Work out the finished part from the listing and answer in its coordinate system (mm). A direction names the side the tool comes from. Give positions to 0.01 mm unless a question says otherwise; leave off trailing zeros. Loops run counter-clockwise (first coordinate to the right, second up) from the corner with the lowest first, then second, coordinate; pieces in that order, holes last.
from build123d import *

# Parameters (mm, degrees)
MODEL_W                 = 10.000078668
MODEL_H                 = 19.99998508
BOSS_EXTRU_1_DEPTH      = 3
ENL_V_MAT_EXTRU_1_DEPTH = 10


with BuildPart() as part:
    # Model → Boss.-Extru.1 (new body)
    with BuildSketch(Plane.XY):
        with BuildLine():
            Line((347.504229039, -990.984743501), (447.504154456, -1164.189847387))
            add(Edge.make_bspline(
                [(447.504154456, -1164.189847387), (453.026125757, -1173.754121475), (449.749150931, -1185.983779814), (440.184876843, -1191.505837242)],
                knots=[1, 1, 1, 1, 2, 2, 2, 2], degree=3))
            Line((440.184876843, -1191.505837242), (447.468153212, -1204.120743383))
            Line((447.468153212, -1204.120743383), (462.904937066, -1204.120743383))
            Line((462.904937066, -1204.120743383), (547.394870334, -1204.120743383))
            Line((547.394870334, -1204.120743383), (562.831654188, -1204.120743383))
            Line((562.831654188, -1204.120743383), (570.114930554, -1191.505837241))
            add(Edge.make_bspline(
                [(570.114930554, -1191.505837241), (560.550656465, -1185.983779815), (557.273681638, -1173.754121476), (562.795652937, -1164.189847387)],
                knots=[7, 7, 7, 7, 8, 8, 8, 8], degree=3))
            Line((562.795652937, -1164.189847387), (662.795578323, -990.984743483))
            add(Edge.make_bspline(
                [(662.795578323, -990.984743483), (668.317549622, -981.420469394), (680.547294088, -978.143580694), (690.111568177, -983.665465865)],
                knots=[9, 9, 9, 9, 10, 10, 10, 10], degree=3))
            Line((690.111568177, -983.665465865), (697.445659701, -970.962451406))
            Line((697.445659701, -970.962451406), (689.778082931, -957.6818667))
            Line((689.778082931, -957.6818667), (647.435103324, -884.341812722))
            Line((647.435103324, -884.341812722), (639.77820635, -871.079314757))
            Line((639.77820635, -871.079314757), (625.092281057, -871.079314757))
            add(Edge.make_bspline(
                [(625.092281057, -871.079314757), (625.092281058, -882.124979905), (616.137961126, -891.079299838), (605.092295979, -891.079299839)],
                knots=[17, 17, 17, 17, 18, 18, 18, 18], degree=3))
            Line((605.092295979, -891.079299839), (405.092272921, -891.079299839))
            add(Edge.make_bspline(
                [(405.092272921, -891.079299839), (394.046607773, -891.07929984), (385.09228784, -882.124979908), (385.092287839, -871.079314761)],
                knots=[19, 19, 19, 19, 20, 20, 20, 20], degree=3))
            Line((385.092287839, -871.079314761), (370.370533553, -871.079314761))
            Line((370.370533553, -871.079314761), (312.778700066, -970.831623929))
            Line((312.778700066, -970.831623929), (320.188239184, -983.665465888))
            add(Edge.make_bspline(
                [(320.188239184, -983.665465888), (329.752513272, -978.143494587), (341.982257738, -981.420469413), (347.504229039, -990.984743501)],
                knots=[23, 23, 23, 23, 24, 24, 24, 24], degree=3))
        make_face()
        Polygon((622.618702509, -993.05007822), (642.608524558, -993.687248628), (642.290025481, -1003.682159653), (622.300031178, -1003.044989244), align=None, mode=Mode.SUBTRACT)
        Polygon((594.878104643, -1072.794736968), (577.611630575, -1062.701812979), (582.658178697, -1054.068575945), (599.924652765, -1064.161499934), align=None, mode=Mode.SUBTRACT)
        Polygon((583.685161648, -902.731560157), (592.474806017, -907.50051971), (582.937059165, -925.079722321), (574.147414796, -920.310848895), align=None, mode=Mode.SUBTRACT)
        Polygon((552.326007751, -1122.752411126), (562.689371739, -1139.857999232), (554.136577686, -1145.039681226), (543.773213697, -1127.93409312), align=None, mode=Mode.SUBTRACT)
        with Locations((505.092198326, -918.785791257)):
            Rectangle(MODEL_W, MODEL_H, mode=Mode.SUBTRACT)
        Polygon((458.493147779, -1123.193383356), (467.045941833, -1128.375065349), (456.682577848, -1145.480653457), (448.129783794, -1140.298971465), align=None, mode=Mode.SUBTRACT)
        Polygon((425.950948052, -902.731560171), (435.488694907, -920.310848907), (426.699050539, -925.079722335), (417.161303684, -907.500519726), align=None, mode=Mode.SUBTRACT)
        Polygon((428.161149075, -1054.509548181), (433.207697199, -1063.142785214), (415.941223133, -1073.235709206), (410.894675009, -1064.602472173), align=None, mode=Mode.SUBTRACT)
        Polygon((388.200625252, -993.491050463), (388.519124331, -1003.485961487), (368.529302282, -1004.123131899), (368.210803204, -994.128220875), align=None, mode=Mode.SUBTRACT)
    extrude(amount=BOSS_EXTRU_1_DEPTH)

    # Esquisse2 → Enlèv. mat.-Extru.1 (cut)
    with BuildSketch(Plane.XY.offset(3)):
        Polygon((377.504209253, -1042.946279151), (407.504189467, -1094.907814801), (450.805469176, -1069.90783129), (420.805488962, -1017.946295639), align=None)
    extrude(amount=-ENL_V_MAT_EXTRU_1_DEPTH, mode=Mode.SUBTRACT)


solid = part.part
Item 1: For faces 1 (the face through (427.22, -1129.06, 1.48)), 2 (the face through (362.294, -1016.602, 1.479)), 3 (the face through (586.37, -1067.82, 1.48)), determine the directions among +Z, -Z, +X, -X, +Y, -Y from which every point of the face is accessible in a straight line to the end or side of a thin tool.
Item 2: Determine the mould class of faces 4 (the face through (502, -1035, 3)), 5 (the face through (421.997, -916.413, 1.479)), 6 (the face through (428.852, -1082.583, 1.521)) for opening direction X: released by +X, released by -X, zero draft, split by the parting line, or undercut.
Item 3: Find section B-B, the plane y = -1029.5. Write down the section's boundary in (x, z), plus the area to 3 significant figures.
Item 4: Consider line 1 (Y direction, x = 506.5, z = 1.4); line 2 (X direction, y = -907, z = 1.75); line 3 (Y direction, x = 441, z = 0.25). Determine where each line is inside the solid, lowest interval first.
Item 5: Find section D-D, the plane x = 483.5. Write down the section's boundary in (y, z).
Item 6: Find section A-A, the plane y = -1135. Write down the section's boundary in (x, z), plus the area to 3 significant figures.
Item 7: Find section C-C, the plane z = 0.75. Give the number of separate pieces and of enclosed holes in the cut face, plus the area to 3 significant figures.
Item 8: Flat-ended cylindrical pins translate along their axes: pin 1 Ø1.5 at (y, z) = (-914.5, 1.5) entering from -X; pin 2 Ø0.9 at (y, z) = (-920, 1.5) entering from +X; pin 3 Ø1.5 at (x, z) = (462.5, 1.5) entering from +Y; pin 4 Ø4 at (x, y) = (383.5, -949) entering from -Z. Find the tip coordinate at first contact, or state that the pin passes through.
Ans:
1. face 1: +Z, -Z, -X
1. face 2: +Z, -Z, -X, -Y
1. face 3: +Z, -Z
2. face 4: zero draft
2. face 5: undercut
2. face 6: released by -X
3. outline: (369.74, 0) - (400.79, 0) - (400.79, 3) - (369.74, 3) - close; (427.48, 0) - (640.56, 0) - (640.56, 3) - (427.48, 3) - close
3. area: 732 mm2
4. line 1: y = -1204.12 to -928.79, -908.79 to -891.08
4. line 2: x = 349.63 to 418.08, 428.27 to 581.37, 591.55 to 660.52
4. line 3: y = -1192.92 to -1191.01, -1152.92 to -1075.57, -1052.92 to -891.08
5. outline: (-1204.12, 0) - (-891.08, 0) - (-891.08, 3) - (-1204.12, 3) - close
6. outline: (430.65, 0) - (451.34, 0) - (451.34, 3) - (430.65, 3) - close; (463.03, 0) - (548.05, 0) - (548.05, 3) - (463.03, 3) - close; (559.75, 0) - (579.65, 0) - (579.65, 3) - (559.75, 3) - close
6. area: 377 mm2
7. separate pieces: 1
7. enclosed holes: 8
7. area: 72,500 mm2
8. pin 1: stops at x = 344.87
8. pin 2: stops at x = 668.28
8. pin 3: stops at y = -891.08
8. pin 4: stops at z = 0
